Can you work these out from the drawing? Everything is in mm from the part's minimum corner. A direction names the side the tool comes from. Round coordinates to 2 decimals unless told otherwise and drop trailing zeros. Write each loop counter-clockwise with the first axis right and the second up, starting at its lowest first coordinate (ties: lowest second). Pieces come first, ordered by that corner, then holes. Notation, with made-up numbers: (72, 1.5) - (96, 1.5) arc R28 cw to (96, 21.5) - close; hole circle Ø7 at (-26.5, 68). An arc over 180 degrees is marked (long way). One line per item, written item: value. Start each with the question number.
(1) I want a section at C-C on y = 50. List the corners of the cut face in (x, z) for me.
(2) I want a section at D-D on x = 29.5. List the corners of the cut face in (y, z) for me, plus the area to 3 significant figures.
(3) I want a section at B-B on z = 47. List the corners of the cut face in (x, y) for me.
(4) On a 3-axis mill with a long thin cutter (end or side, diameter ignored), from which of +Z, -Z, +X, -X, +Y, -Y can I reach the whole of each face in a straight line? I mean the marked faces 1, 2, 3 and 4. Say none if no direction works.
(5) Thinking about a two-plate mould opening in X: for the marked faces 5, 6 and 7, which applies, +X half, -X half, draft (parallel to the pull), parting line (faces both ways), or undercut?
(6) I want a section at A-A on z = 31. List the corners of the cut face in (x, y) for me.
(7) If I drill on L1, parallel to X at y = 3, z = 5; L2, parallel to Y at x = 6.4, z = 31; L3, parallel to Z at x = 21.5, y = 1.05, over which ranges is the centre line in solid material (lowest first)? Write a range as from..to.
(8) I'm going to push flat-ended pins straight in: pin 1 Ø12.5 at (y, z) = (31, 39) entering from -X; pin 2 Ø2 at (x, y) = (51, 52.5) entering from -Z; pin 3 Ø8 at (x, y) = (31, 20) entering from +Z. Where does each tip first touch, or does it pass through?
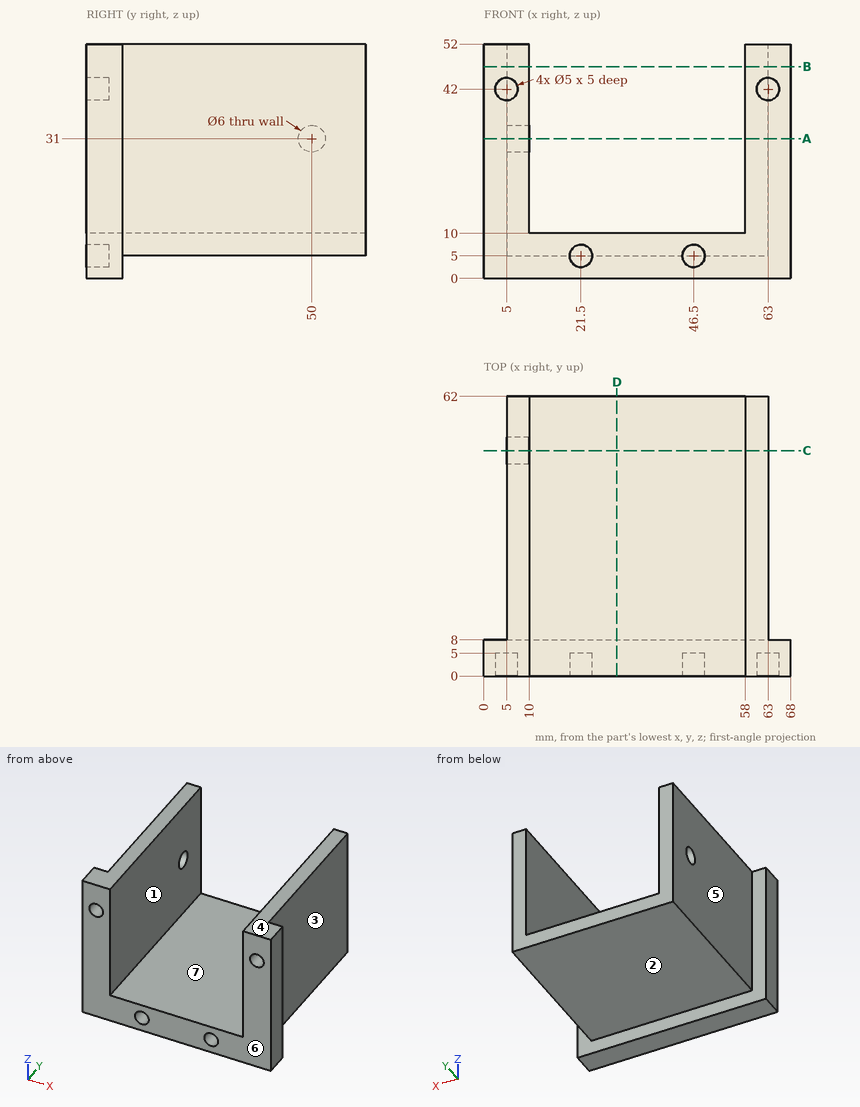
Established:
1. outline: (5, 5) - (63, 5) - (63, 52) - (58, 52) - (58, 10) - (10, 10) - (10, 28) - (5, 28) - close; (5, 34) - (10, 34) - (10, 52) - (5, 52) - close
2. outline: (0, 0) - (8, 0) - (8, 5) - (62, 5) - (62, 10) - (0, 10) - close
2. area: 350 mm2
3. outline: (0, 0) - (10, 0) - (10, 62) - (5, 62) - (5, 8) - (0, 8) - close; (58, 0) - (68, 0) - (68, 8) - (63, 8) - (63, 62) - (58, 62) - close
4. face 1: +Z, +Y, -Y
4. face 2: -Z, +X, -X, +Y
4. face 3: +Z, -Z, +X, +Y
4. face 4: +Z, +X, -X, +Y, -Y
5. face 5: -X half
5. face 6: draft
5. face 7: undercut
6. outline: (0, 0) - (10, 0) - (10, 47) - (5, 47) - (5, 8) - (0, 8) - close; (5, 53) - (10, 53) - (10, 62) - (5, 62) - close; (58, 0) - (68, 0) - (68, 8) - (63, 8) - (63, 62) - (58, 62) - close
7. L1: 0..19, 24..44, 49..68
7. L2: 0..47, 53..62
7. L3: 0..2.5, 7.5..10
8. pin 1: x = 5
8. pin 2: z = 5
8. pin 3: z = 10
